Verification items for the finished model (mm, model axes). A direction names the side the tool comes from. Round coordinates to 2 decimals unless told otherwise and drop trailing zeros. Write each loop counter-clockwise with the first axis right and the second up, starting at its lowest first coordinate (ties: lowest second). Pieces come first, ordered by that corner, then holes. Notation, with made-up numbers: (39.5, -6.5) - (81.5, -6.5) arc R22 cw to (81.5, 22.5) - close; hole circle Ø2 at (85, 23.5). An arc over 180 degrees is marked (long way). Answer as a JSON object with one key per item and string values.
```python
from build123d import *

# Parameters (mm, degrees)
PAD_DEPTH   = 6
FILLET_R    = 2.5
FILLET001_R = 1


with BuildPart() as part:
    # Sketch → Pad (new body)
    with BuildSketch(Plane.XY):
        Polygon((0, 7), (-2, 7), (-2, 3), (-3.2, 3), (-3.2, 6), (-5.2, 6), (-5.2, 0), (-5.2, -6), (-3.2, -6), (-3.2, -3), (-2, -3), (-2, -7), (0, -7), (2, -7), (2, -3), (3.2, -3), (3.2, -6), (5.2, -6), (5.2, 0), (5.2, 6), (3.2, 6), (3.2, 3), (2, 3), (2, 7), align=None)
    extrude(amount=PAD_DEPTH)

    # Fillet
    fillet_edges = [part.edges().sort_by_distance(p)[0] for p in [
        (-4.2, 6, 6),
        (-4.2, 6, 0),
        (-4.2, -6, 0),
        (-4.2, -6, 6),
        (4.2, -6, 0),
        (4.2, -6, 6),
        (4.2, 6, 6),
        (4.2, 6, 0),
        (0, 7, 0),
        (0, -7, 0),
        (0, -7, 6),
        (0, 7, 6),
    ]]
    fillet(fillet_edges, radius=FILLET_R)

    # Fillet001
    fillet001_edges = [part.edges().sort_by_distance(p)[0] for p in [
        (-5.2, 6, 3),
        (-5.2, 5.267767, 0.732233),
        (-5.2, 5.267767, 5.267767),
        (-5.2, 0, 0),
        (-5.2, 0, 6),
        (-5.2, -5.267767, 0.732233),
        (-5.2, -5.267767, 5.267767),
        (-5.2, -6, 3),
        (5.2, -6, 3),
        (5.2, -5.267767, 0.732233),
        (5.2, -5.267767, 5.267767),
        (5.2, 0, 0),
        (5.2, 0, 6),
        (5.2, 5.267767, 0.732233),
        (5.2, 5.267767, 5.267767),
        (5.2, 6, 3),
    ]]
    fillet(fillet001_edges, radius=FILLET001_R)


solid = part.part
```
Q1. Gauge pin test, flat ends, axial feed: P1, Ø2, axis at x = 2, z = 1.5, coming from the -Y side; P2, Ø0.8, axis at x = -4, z = 3, coming from the +Y side; P3, Ø0.5, axis at x = 3.5, z = 3, coming from the -Y side; P4, Ø1, axis at x = -3, z = 1, coming from the -Y side. Record the tip position at first contact, or that the pin passes through.
Geometry check:
{"P1": "stops at y = -7", "P2": "stops at y = 6", "P3": "stops at y = -6", "P4": "stops at y = -5.77"}
Q2. Release check for a two-part mould opening along X. For faces 6 (the flat face through (3, 3, 3)), 7 (the flat face through (-5.2, 0, 3)), 8 (the cylindrical face through (0.028, -6.287, 0.752)) record: released by +X, released by -X, zero draft, split by the parting line, or undercut.
Geometry check:
{"face 6": "undercut", "face 7": "released by -X", "face 8": "zero draft"}
Q3. Set-up check for faces 1 (the cylindrical face through (-3.707, 5.287, 5.248)), 2 (the cylindrical face through (3.693, 5.287, 5.248)), 3 (the flat face through (4, 6, 3)), 4 (the cylindrical face through (3.707, -5.287, 0.752)), 5 (the flat face through (3.2, -4, 3)): record each of +Z, -Z, +X, -X, +Y, -Y from which the full face is reachable in a straight line by a thin tool's end or side.
Geometry check:
{"face 1": "+Z, -X, +Y", "face 2": "+Z, +X, +Y", "face 3": "+Z, -Z, +X, +Y", "face 4": "-Z, +X, -Y", "face 5": "+Z, -Z, -Y"}
Q4. Section check A-A, the plane x = 1.5. Record the cut outline in (y, z).
Geometry check:
{"outline": "(-7, 2.5) arc R2.5 ccw to (-4.5, 0) - (4.5, 0) arc R2.5 ccw to (7, 2.5) - (7, 3.5) arc R2.5 ccw to (4.5, 6) - (-4.5, 6) arc R2.5 ccw to (-7, 3.5) - close"}
Q5. Section check C-C, the plane x = -3.75. Record the cut outline in (y, z).
Geometry check:
{"outline": "(-6, 2.5) arc R2.5 ccw to (-3.5, 0) - (3.5, 0) arc R2.5 ccw to (6, 2.5) - (6, 3.5) arc R2.5 ccw to (3.5, 6) - (-3.5, 6) arc R2.5 ccw to (-6, 3.5) - close"}
Q6. Material ranges on line 1 along X through (y, z) = (-4.5, 2.75); line 2 along Y through (x, z) = (2.5, 2.5); line 3 along Y through (x, z) = (4, 3.45), recorded low to high. Write a range as [from, to].
Geometry check:
{"line 1": "x = [-5.2, -3.2], [-2, 2], [3.2, 5.2]", "line 2": "y = [-3, 3]", "line 3": "y = [-6, 6]"}
Q7. Section check B-B, the plane y = -4.25. State how many separate pieces and enclosed holes the cut face has, then the cut area to 3 significant figures.
Geometry check:
{"separate pieces": "3", "enclosed holes": "0", "area": "46.2 mm2"}
